The model under review builds one solid part; all positions refer to its coordinate system, in mm. Coordinates: 2 decimals unless noted, no trailing zeros. Order: outer loops, then holes, each group sorted by start corner. A loop starts at its lowest first (then second) coordinate and runs counter-clockwise, first axis right, second up. Notation, with made-up numbers: (22.5, -32) -> (53.5, -32) arc R18 ccw to (53.5, -7) -> close; hole circle Ø5 at (58, 48.25). An arc over 180 degrees is marked (long way). Use one line per item in the form item = value. Start each with the question number.
(1) Take a section at C-C (y = 2.2). State the section outline as (x, z) points.
(2) Insertion check: pin 1 Ø1 at (y, z) = (2, 6.5) entering from +X; pin 2 Ø1.5 at (x, y) = (2.5, 1.5) entering from -Z. Each pin has a flat end and moves straight along its axis. Give the tip position at first contact, or say it passes through.
(3) Mouldability with a two-part tool opening along X and no side actions: class faces 1 (the flat face through (-5, 0, -5)), 2 (the cylindrical face through (5.676, 1.43, 3.619)), 3 (the cylindrical face through (5.78, 2.19, 7.54)) as +X half, -X half, draft (parallel to the pull), parting line (faces both ways), or undercut.
(4) Take a section at D-D (y = 0.45). State the section outline as (x, z) points.
(5) Wall thickness on line 1 along X through (y, z) = (1.7, 0); line 2 along Z through (x, y) = (1.5, 1.2); line 3 along X through (y, z) = (1.65, 5.75): over which ranges is each line inside the solid? List them lowest first.
```python
from build123d import *

# Parameters (mm, degrees)
SKETCH1_R           = 11
SKETCH1_R_2         = 6.731
BOSS_EXTRUDE1_DEPTH = 1.5
CHAMFER1_SIZE       = 1.5
SKETCH2_R           = 9.5
SKETCH2_R_2         = 6.731
BOSS_EXTRUDE2_DEPTH = 1.4


with BuildPart() as part:
    # Sketch1 → Boss-Extrude1 (new body)
    with BuildSketch(Plane(origin=(0, 0, 0), x_dir=(1, 0, 0), z_dir=(0, 1, 0))):
        with Locations(Location((0, 0, 0), (0, 0, 270))):
            Circle(SKETCH1_R)
        with Locations(Location((0, 0, 0), (0, 0, 270))):
            Circle(SKETCH1_R_2, mode=Mode.SUBTRACT)
    extrude(amount=BOSS_EXTRUDE1_DEPTH)

    # Chamfer1
    chamfer1_edges = [part.edges().sort_by_distance(p)[0] for p in [
        (0, 1.5, -11),
    ]]
    chamfer(chamfer1_edges, length=CHAMFER1_SIZE - 0.0001)  # a hair under: the kernel refuses the full size

    # Sketch2 → Boss-Extrude2 (add)
    with BuildSketch(Plane(origin=(0, 1.5, 0), x_dir=(1, 0, 0), z_dir=(0, 1, 0))):
        with Locations(Location((0, 0, 0), (0, 0, 90))):
            Circle(SKETCH2_R)
        with Locations(Location((0, 0, 0), (0, 0, 270))):
            Circle(SKETCH2_R_2, mode=Mode.SUBTRACT)
    extrude(amount=BOSS_EXTRUDE2_DEPTH)


solid = part.part
```
Findings:
q1.outline = circle Ø19 at (0, 0); hole circle Ø13.46 at (0, 0)
q2.pin_1 = 7.37
q2.pin_2 = -9.96
q3.face_1 = draft
q3.face_2 = undercut
q3.face_3 = parting line
q4.outline = circle Ø21.1 at (0, 0); hole circle Ø13.46 at (0, 0)
q5.line_1 = -9.5 to -6.73, 6.73 to 9.5
q5.line_2 = -9.68 to -6.56, 6.56 to 9.68
q5.line_3 = -7.56 to -3.5, 3.5 to 7.56
